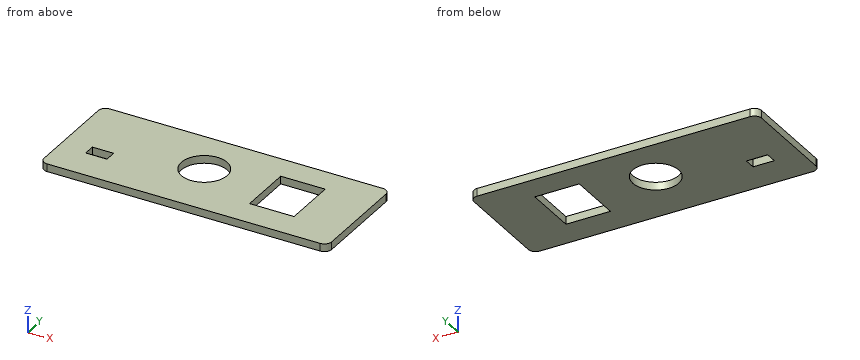
Autodesk Inventor part; units mm, degrees
ref_plane "YZ Plane" through (0, 0, 0) normal (1, 0, 0) x (0, 1, 0)
ref_plane "XZ Plane" through (0, 0, 0) normal (0, 1, 0) x (-1, 0, 0)
ref_plane "XY Plane" through (0, 0, 0) normal (0, 0, 1) x (1, 0, 0)
sketch "Sketch1" plane through (0, 0, 0) normal (0, 0, 1) x (1, 0, 0)
  line L0 (-29.75, -11.25) -> (29.75, -11.25)
  line L1 (29.75, -11.25) -> (29.75, 11.25)
  line L2 (29.75, 11.25) -> (-29.75, 11.25)
  line L3 (-29.75, 11.25) -> (-29.75, -11.25)
  line L4 (-29.75, -11.25) -> (29.75, 11.25) construction
  line L5 (29.75, -11.25) -> (-29.75, 11.25) construction
  point P0 (0, 0)
  dimension "d0" = 59.5
  dimension "d1" = 22.5
extrude "Extrusion1" add sketch "Sketch1" against normal blind 1.6
fillet "Fillet1" radius 1.5 4 edges at (29.75, 11.25, -0.8) (29.75, -11.25, -0.8) (-29.75, 11.25, -0.8) (-29.75, -11.25, -0.8)
sketch "Sketch2" plane through (0, 0, 0) normal (0, 0, 1) x (1, 0, 0)
  circle A0 centre (-2.949, 1.26) radius 4.75
  line L0 (-28.25, -11.25) -> (28.25, -11.25)
  line L1 (-29.75, 9.75) -> (-29.75, -9.75)
  line L2 (-24.199, -4.44) -> (-19.799, -4.44)
  line L3 (-19.799, -4.44) -> (-19.799, -2.04)
  line L4 (-19.799, -2.04) -> (-24.199, -2.04)
  line L5 (-24.199, -2.04) -> (-24.199, -4.44)
  line L6 (-24.199, -4.44) -> (-19.799, -2.04) construction
  line L7 (-19.799, -4.44) -> (-24.199, -2.04) construction
  point P0 (0, 0)
  point P1 (-28.349, -5.24)
  point P2 (-21.999, -3.24)
  dimension "d5" = 9.5
  dimension "d15" = 12.51
  dimension "d16" = 26.801
  dimension "d17" = 6.01
  dimension "d18" = 1.401
  dimension "d19" = 4.4
  dimension "d20" = 2.4
  dimension "d21" = 6.35
  dimension "d22" = 2
extrude "Extrusion2" cut sketch "Sketch2" against normal through all
sketch "Sketch4" plane through (0, 0, 0) normal (0, 0, 1) x (1, 0, 0)
  line L0 (-28.25, -11.25) -> (28.25, -11.25)
  line L1 (-29.75, 9.75) -> (-29.75, -9.75)
  line L2 (10.231, -5.34) -> (19.431, -5.34)
  line L3 (19.431, -5.34) -> (19.431, 5.86)
  line L4 (19.431, 5.86) -> (10.231, 5.86)
  line L5 (10.231, 5.86) -> (10.231, -5.34)
  line L6 (10.231, -5.34) -> (19.431, 5.86) construction
  line L7 (19.431, -5.34) -> (10.231, 5.86) construction
  point P0 (0, 0)
  point P1 (-28.349, -5.24)
  point P2 (14.831, 0.26)
  dimension "d23" = 6.01
  dimension "d24" = 1.401
  dimension "d25" = 9.2
  dimension "d26" = 11.2
  dimension "d28" = 43.18
  dimension "d29" = 0.1
extrude "Extrusion4" cut sketch "Sketch4" against normal through all
properties part number "rearPlate_jack"
Input: part model. Units: mm. Frame: model coordinates. Coordinates: 2 decimals unless noted, no trailing zeros. Write each loop counter-clockwise with the first axis right and the second up, starting at its lowest first coordinate (ties: lowest second). Pieces come first, ordered by that corner, then holes. Notation, with made-up numbers: (18, 77.25) -> (70, 77.25) arc R15 ccw to (70, 98.25) -> close; hole circle Ø4 at (27, -6). An arc over 180 degrees is marked (long way). Write each question's results on one line, items separated by ' | '.
Item 1: Section query C-C on x = -5. Return loops of the section in (y, z).
Conclusion:
outline: (-11.25, -1.6) -> (-3.02, -1.6) -> (-3.02, 0) -> (-11.25, 0) -> close; (5.54, -1.6) -> (11.25, -1.6) -> (11.25, 0) -> (5.54, 0) -> close
Item 2: Pin query (flat end, axial travel): pin 1 Ø7.5 at (x, y) = (-2.949, 1.26) entering from +Z. Return the tip coordinate at first contact, or that it passes through.
Conclusion:
pin 1: passes through
Item 3: Section query B-B on y = 1.26. Return loops of the section in (x, z), plus the area to 3 significant figures.
Conclusion:
outline: (-29.75, -1.6) -> (-7.7, -1.6) -> (-7.7, 0) -> (-29.75, 0) -> close; (1.8, -1.6) -> (10.23, -1.6) -> (10.23, 0) -> (1.8, 0) -> close; (19.43, -1.6) -> (29.75, -1.6) -> (29.75, 0) -> (19.43, 0) -> close | area: 65.3 mm^2
Item 4: Section query A-A on z = -0.3. Return loops of the section in (x, y).
Conclusion:
outline: (-29.75, -9.75) arc R1.5 ccw to (-28.25, -11.25) -> (28.25, -11.25) arc R1.5 ccw to (29.75, -9.75) -> (29.75, 9.75) arc R1.5 ccw to (28.25, 11.25) -> (-28.25, 11.25) arc R1.5 ccw to (-29.75, 9.75) -> close; hole (-24.2, -4.44) -> (-19.8, -4.44) -> (-19.8, -2.04) -> (-24.2, -2.04) -> close; hole circle Ø9.5 at (-2.95, 1.26); hole (10.23, -5.34) -> (19.43, -5.34) -> (19.43, 5.86) -> (10.23, 5.86) -> close
Item 5: Material intervals for probe 1 along X at (y, z) = (-4.25, -0.6); probe 2 along X at (y, z) = (1, -0.8); probe 3 along Y at (x, z) = (-23, -1.5), sorted ascending.
Conclusion:
probe 1: x = -29.75 to -24.2, -19.8 to 10.23, 19.43 to 29.75 | probe 2: x = -29.75 to -7.69, 1.79 to 10.23, 19.43 to 29.75 | probe 3: y = -11.25 to -4.44, -2.04 to 11.25
